Verification items for this drawing (mm, ordinates from the low corner). A direction names the side the tool comes from. Give positions to 0.01 mm unless a question says otherwise; leave off trailing zeros. Write each loop counter-clockwise with the first axis right and the second up, starting at its lowest first coordinate (ties: lowest second). Pieces come first, ordered by that corner, then holes. Notation, with made-up numbers: (-27, 6.25) -> (-16, 6.25) arc R26 cw to (-16, 27.25) -> close; hole circle Ø5 at (60.25, 3). An arc over 180 degrees is marked (long way). Use one line per item in the form item = value. Start each with the question number.
(1) Depth check by flat-ended pin: pin 1 Ø1.8 at (y, z) = (1.5, 12) entering from +X; pin 2 Ø4 at (x, z) = (34.5, 22) entering from -Y; pin 3 Ø2.5 at (x, z) = (75, 58) entering from +Y. Enter the tip coordinate at first touch or a pass-through.
(2) Section check D-D, the plane x = 47. Record the cut outline in (y, z), plus the area to 3 significant figures.
(3) Section check B-B, the plane z = 45.5. Record the cut outline in (x, y).
(4) Set-up check for the marked faces 1, 2, 3 and 4: record each of +Z, -Z, +X, -X, +Y, -Y from which the full face is reachable in a straight line by a thin tool's end or side.
(5) Release check for a two-part mould opening along Y. For the marked faces 5, 6 and 7 record: pulls with the +Y half, pulls with the -Y half, needs draft (parallel to the pull), parting line crosses it, or undercut.
(6) Scan lines: L1, parallel to Y at x = 5, z = 5; L2, parallel to Y at x = 5, z = 22; L3, parallel to Y at x = 15, z = 24.25. Record each from-to range of solid material in increasing order.
(7) Section check A-A, the plane z = 56.25. Record the cut outline in (x, y), plus the area to 3 significant figures.
(8) Section check C-C, the plane z = 5. Record the cut outline in (x, y).
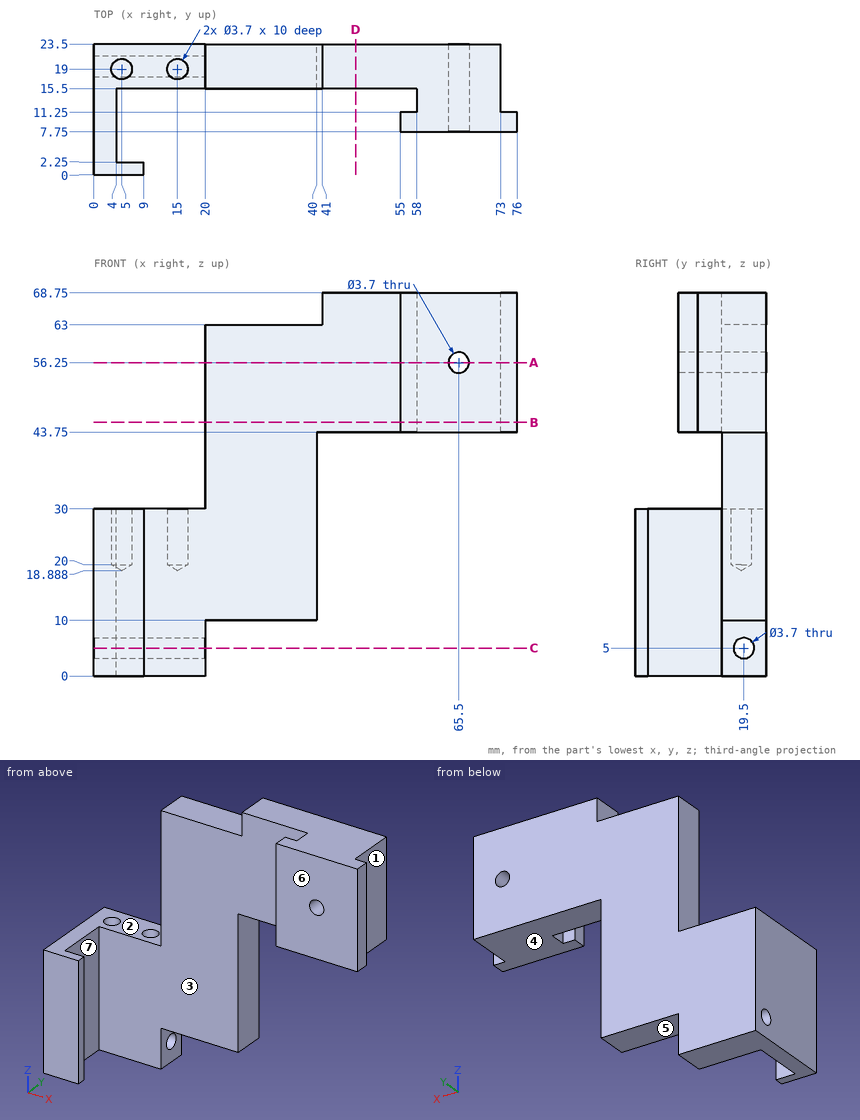
Completed:
q1.pin_1 = 9
q1.pin_2 = 15.5
q1.pin_3 = 11.25
q2.outline = (15.5, 43.75) -> (23.5, 43.75) -> (23.5, 68.75) -> (15.5, 68.75) -> close
q2.area = 200 mm²
q3.outline = (20, 15.5) -> (58, 15.5) -> (58, 11.25) -> (55, 11.25) -> (55, 7.75) -> (76, 7.75) -> (76, 11.25) -> (73, 11.25) -> (73, 23.5) -> (20, 23.5) -> close
q4.face_1 = +Z, -Z, +X, +Y
q4.face_2 = +Z, -X, +Y, -Y
q4.face_3 = +Z, -Z
q4.face_4 = -Z, +X, +Y, -Y
q5.face_5 = needs draft
q5.face_6 = pulls with the -Y half
q5.face_7 = undercut
q6.L1 = 0 to 2.25, 15.5 to 17.65, 21.35 to 23.5
q6.L2 = 0 to 2.25, 15.5 to 17.15, 20.85 to 23.5
q6.L3 = 15.5 to 17.15, 20.85 to 23.5
q7.outline = (20, 15.5) -> (58, 15.5) -> (58, 11.25) -> (55, 11.25) -> (55, 7.75) -> (63.65, 7.75) -> (63.65, 23.5) -> (20, 23.5) -> close; (67.35, 7.75) -> (76, 7.75) -> (76, 11.25) -> (73, 11.25) -> (73, 23.5) -> (67.35, 23.5) -> close
q7.area = 503 mm²
q8.outline = (0, 0) -> (9, 0) -> (9, 2.25) -> (4, 2.25) -> (4, 15.5) -> (20, 15.5) -> (20, 17.65) -> (0, 17.65) -> close; (0, 21.35) -> (20, 21.35) -> (20, 23.5) -> (0, 23.5) -> close
